Input: part model. Units: mm. Frame: model coordinates. A direction names the side the tool comes from. Give positions to 0.01 mm unless a question says otherwise; leave off trailing zeros. Order: outer loops, then holes, each group sorted by start corner. A loop starts at its lowest first (then second) coordinate and runs counter-clockwise, first axis right, second up. Notation, with made-up numbers: M -5,59 L 8,59 A16 cw 8,74 Z; hole C 61.5,14.5 d1. An arc over 180 degrees is marked long. Use a Markdown table: item, result.
from build123d import *

# Parameters (mm, degrees)
SKETCH1_R           = 23
SKETCH1_R_2         = 21
EXTRUDE_THIN1_DEPTH = 27
SKETCH2_R           = 19
SKETCH2_R_2         = 17
EXTRUDE_THIN2_DEPTH = 23
SKETCH3_R           = 21
BOSS_EXTRUDE1_DEPTH = 6
BOSS_EXTRUDE1_TAPER = 34
SKETCH4_R           = 23
BOSS_EXTRUDE2_DEPTH = 6
BOSS_EXTRUDE2_TAPER = 34


with BuildPart() as part:
    # Sketch1 → Extrude-Thin1 (new body)
    with BuildSketch(Plane(origin=(0, 0, 0), x_dir=(1, 0, 0), z_dir=(0, 1, 0))):
        Circle(SKETCH1_R)
        Circle(SKETCH1_R_2, mode=Mode.SUBTRACT)
    extrude(amount=EXTRUDE_THIN1_DEPTH)



with BuildPart() as body_2:
    # Sketch2 → Extrude-Thin2 (new body)
    with BuildSketch(Plane(origin=(0, 0, 0), x_dir=(1, 0, 0), z_dir=(0, 1, 0))):
        Circle(SKETCH2_R)
        Circle(SKETCH2_R_2, mode=Mode.SUBTRACT)
    extrude(amount=EXTRUDE_THIN2_DEPTH)


with BuildPart() as body_2_1:
    # Move Face1: read off the stored shape, not the designer's step
    # Move Face1: moved
    add(body_2.part.moved(Location((0, 33, 0))))


with BuildPart() as body_3:
    # Sketch3 → Boss-Extrude1 (new body)
    with BuildSketch(Plane(origin=(0, 27, 0), x_dir=(1, 0, 0), z_dir=(0, 1, 0))):
        with Locations(Location((0, 0, 0), (0, 0, 270))):
            Circle(SKETCH3_R)
    extrude(amount=BOSS_EXTRUDE1_DEPTH, taper=BOSS_EXTRUDE1_TAPER)


with BuildPart() as part_1:
    add(part.part)

    add(body_2_1.part)  # Boss-Extrude2 merges body 2

    add(body_3.part)  # Boss-Extrude2 merges body 3
    # Sketch4 → Boss-Extrude2 (add)
    with BuildSketch(Plane(origin=(0, 27, 0), x_dir=(1, 0, 0), z_dir=(0, 1, 0))):
        Circle(SKETCH4_R)
    extrude(amount=BOSS_EXTRUDE2_DEPTH, taper=BOSS_EXTRUDE2_TAPER)


solid = part_1.part
1) Material intervals for line 1 (X direction, y = 42, z = 0); line 2 (Z direction, x = 0, y = 7), sorted ascending. Write a range as from..to.
Response values:
| item | result |
|---|---|
| line 1 | x = -19..-17, 17..19 |
| line 2 | z = -23..-21, 21..23 |
2) Cut plane B-B on x = 0. Return loops of the section in (y, z), and give its area (3 significant figures).
Response values:
| item | result |
|---|---|
| outline | M 0,-23 L 27,-23 L 33,-18.95 L 33,-19 L 56,-19 L 56,-17 L 33,-17 L 33,17 L 56,17 L 56,19 L 33,19 L 33,18.95 L 27,23 L 0,23 L 0,21 L 27,21 L 27,-21 L 0,-21 Z |
| area | 452 mm² |
3) Cut plane D-D on y = 29. Return loops of the section in (x, z), and give its area (3 significant figures).
Response values:
| item | result |
|---|---|
| outline | C 0,0 d43.3 |
| area | 1,470 mm² |
4) First-contact query: pin 1 Ø1 at (x, y) = (13.5, 30.5) entering from -Z; pin 2 Ø4 at (y, z) = (31, -17) entering from +X; pin 3 Ø12 at (x, y) = (0, 28.5) entering from -Z. Flat tips, straight axial feed; report the tip coordinate or a pass-through.
Response values:
| item | result |
|---|---|
| pin 1 | stops at z = -16.22 |
| pin 2 | stops at x = 14.46 |
| pin 3 | stops at z = -23 |
5) Cut plane A-A on y = 43. Return loops of the section in (x, z), and give its area (3 significant figures).
Response values:
| item | result |
|---|---|
| outline | C 0,0 d38; hole C 0,0 d34 |
| area | 226 mm² |
6) Reachability of faces 1 (the face through (-2.994, 13.311, -22.804)), 2 (the face through (9.139, 44.339, -14.334)), 3 (the face through (0, 27, 0)) from +Z, -Z, +X, -X, +Y, -Y: full face, straight path, thin tool, end or side. Return the list, or none.
Response values:
| item | result |
|---|---|
| face 1 | +Y, -Y |
| face 2 | +Y |
| face 3 | -Y |
7) Cut plane C-C on y = 20. Return loops of the section in (x, z).
Response values:
| item | result |
|---|---|
| outline | C 0,0 d46; hole C 0,0 d42 |
8) Mould query, pull axis X, two halves, no side actions, for faces 4 (the face through (20.03, 13.31, -6.31)), 5 (the face through (8.767, 44.339, 16.856)), 6 (the face through (0, 33, 0)), 7 (the face through (-14, 56, 10)). Classes: released by +X, released by -X, zero draft, split by the parting line, or undercut.
Response values:
| item | result |
|---|---|
| face 4 | undercut |
| face 5 | split by the parting line |
| face 6 | undercut |
| face 7 | zero draft |
